Part model, mm, in its own coordinate system. A direction names the side the tool comes from. Give positions to 0.01 mm unless a question says otherwise; leave off trailing zeros. Write each loop counter-clockwise with the first axis right and the second up, starting at its lowest first coordinate (ties: lowest second). Pieces come first, ordered by that corner, then holes.
from build123d import *

# Parameters (mm, degrees)
T_LE_DE_BASE_PLI_E1_DEPTH = 30
ESQUISSE13_R              = 4.5
ESQUISSE13_R_2            = 0.8
ENL_V_MAT_EXTRU_2_DEPTH   = 72.281133549


# Sheet-metal steps are written as plain solids
with BuildPart() as part:
    # Esquisse1 → Tôle de base pliée1 (new body)
    with BuildSketch(Plane.XY):
        with BuildLine():
            Line((-50, 20.5), (-1.4732, 20.5))
            ThreePointArc((-1.4732, 20.5), (-0.43149029, 20.06850971), (0, 19.0268))
            Line((0, 19.0268), (0, -19.0268))
            ThreePointArc((0, -19.0268), (-0.43149029, -20.06850971), (-1.4732, -20.5))
            Line((-1.4732, -20.5), (-50, -20.5))
            Line((-50, -20.5), (-50, -19.7634))
            Line((-50, -19.7634), (-1.4732, -19.7634))
            ThreePointArc((-1.4732, -19.7634), (-0.952345145, -19.547654855), (-0.7366, -19.0268))
            Line((-0.7366, -19.0268), (-0.7366, 19.0268))
            ThreePointArc((-0.7366, 19.0268), (-0.952345145, 19.547654855), (-1.4732, 19.7634))
            Line((-1.4732, 19.7634), (-50, 19.7634))
            Line((-50, 19.7634), (-50, 20.5))
        make_face()
    extrude(amount=T_LE_DE_BASE_PLI_E1_DEPTH)

    # Esquisse13 → Enlèv. mat.-Extru.2 (cut, through all)
    with BuildSketch(Plane.XZ.offset(20.5)):
        with BuildLine():
            ThreePointArc((-46.549919552, 15), (-44.463516741, 20.940418901), (-39.120745506, 24.271552182))
            Line((-39.120745506, 24.271552182), (-13.4732, 30))
            Line((-13.4732, 30), (-50, 30))
            Line((-50, 30), (-50, 15))
            Line((-50, 15), (-46.549919552, 15))
        make_face()
        with BuildLine():
            Line((-13.4732, 0), (-39.120745506, 5.728447818))
            ThreePointArc((-39.120745506, 5.728447818), (-44.463516741, 9.059581099), (-46.549919552, 15))
            Line((-46.549919552, 15), (-50, 15))
            Line((-50, 15), (-50, 0))
            Line((-50, 0), (-13.4732, 0))
        make_face()
        with Locations((-37.049919552, 15)):
            Circle(ESQUISSE13_R)
        with Locations((-30.049919552, 16.017866465)):
            Circle(ESQUISSE13_R_2)
        with Locations((-32.819912364, 20.669487748)):
            Circle(ESQUISSE13_R_2)
        with Locations((-38.067786017, 22)):
            Circle(ESQUISSE13_R_2)
        with Locations((-42.7194073, 19.230007189)):
            Circle(ESQUISSE13_R_2)
        with Locations((-44.049919552, 13.982133535)):
            Circle(ESQUISSE13_R_2)
        with Locations((-41.279926741, 9.330512252)):
            Circle(ESQUISSE13_R_2)
        with Locations((-36.032053088, 8)):
            Circle(ESQUISSE13_R_2)
        with Locations((-31.380431805, 10.769992811)):
            Circle(ESQUISSE13_R_2)
    extrude(amount=-ENL_V_MAT_EXTRU_2_DEPTH, mode=Mode.SUBTRACT)


solid = part.part
1) Saw through at A-A (x = -25). Write the cut outline in (y, z).
Check result:
outline: (-20.5, 2.57) - (-19.76, 2.57) - (-19.76, 27.43) - (-20.5, 27.43) - close; (19.76, 2.57) - (20.5, 2.57) - (20.5, 27.43) - (19.76, 27.43) - close
2) Flat gauge pin, fed straight in: P1, Ø3, axis at y = 10.5, z = 20.5, coming from the -X side. Where does the tip first touch, or does it go through?
Check result:
P1: stops at x = -0.74
3) 3-axis set-ups, long thin cutter, end or side, ignore diameter. For faces 1 (the flat face through (-19, 19.763, 15)), 2 (the flat face through (-0.2, 6.2, 0)): which of +Z, -Z, +X, -X, +Y, -Y reach the whole face in a straight line?
Check result:
face 1: +Z, -Z, -X
face 2: -Z, +X, -X, +Y, -Y
4) Saw through at C-C (y = -13.5). Write the cut outline in (x, z).
Check result:
outline: (-0.74, 0) - (0, 0) - (0, 30) - (-0.74, 30) - close
5) Saw through at B-B (z = 27.75). Write the cut outline in (x, y).
Check result:
outline: (-23.55, -20.5) - (-1.47, -20.5) arc R1.47 ccw to (0, -19.03) - (0, 19.03) arc R1.47 ccw to (-1.47, 20.5) - (-23.55, 20.5) - (-23.55, 19.76) - (-1.47, 19.76) arc R0.74 cw to (-0.74, 19.03) - (-0.74, -19.03) arc R0.74 cw to (-1.47, -19.76) - (-23.55, -19.76) - close
6) Mould opens along X. For faces 3 (the cylindrical face through (-35.27, -20.14, 8.24)), 4 (the flat face through (-0.737, 0, 15)), 5 (the cylindrical face through (-0.443, 20.08, 14.79)) say: +X half, -X half, draft (parallel to the pull), parting line (faces both ways), or undercut.
Check result:
face 3: undercut
face 4: -X half
face 5: +X half
7) Drill centre lines: L1, parallel to Y at x = -21.5, z = 14.5; L2, parallel to X at y = 9.5, z = 20.5; L3, parallel to X at y = 19.5, z = 3.75. Where is each one in solid material? Low to high.
Check result:
L1: y = -20.5 to -19.76, 19.76 to 20.5
L2: x = -0.74 to 0
L3: x = -0.91 to -0.08
8) Saw through at D-D (x = -14.5). Write the cut outline in (y, z).
Check result:
outline: (-20.5, 0.23) - (-19.76, 0.23) - (-19.76, 29.77) - (-20.5, 29.77) - close; (19.76, 0.23) - (20.5, 0.23) - (20.5, 29.77) - (19.76, 29.77) - close
